from build123d import *

# Parameters (mm, degrees)
SCHIZZO13_R                  = 1.5
SCHIZZO13_R_2                = 2.75
SCHIZZO13_R_3                = 1.25
ESTRUSIONE_ESTRUSIONE2_DEPTH = 6


with BuildPart() as part:
    # Schizzo13 → Estrusione-Estrusione2 (new body)
    with BuildSketch(Plane.XY):
        with BuildLine():
            Line((9.919241786, 0), (24.201199756, 0))
            Line((24.201199756, 0), (34.201199756, 10))
            Line((34.201199756, 10), (34.28195797, 30))
            Line((34.28195797, 30), (57.017366293, 53.192694567))
            Line((57.017366293, 53.192694567), (83.745372993, 53.192694567))
            Line((83.745372993, 53.192694567), (107.404551383, 30))
            Line((107.404551383, 30), (107.404551383, 10))
            Line((107.404551383, 10), (117.404551383, 0))
            Line((117.404551383, 0), (232.595448617, 0))
            Line((232.595448617, 0), (242.595448617, 10))
            Line((242.595448617, 10), (242.595448617, 30))
            Line((242.595448617, 30), (266.254627007, 53.192694567))
            Line((266.254627007, 53.192694567), (292.982633707, 53.192694567))
            Line((292.982633707, 53.192694567), (315.71804203, 30))
            Line((315.71804203, 30), (315.71804203, 10))
            Line((315.71804203, 10), (325.71804203, 0))
            Line((325.71804203, 0), (340, 0))
            Line((340, 0), (350, 10))
            Line((350, 10), (350.080758214, 70.5))
            Line((350.080758214, 70.5), (293, 124.388863529))
            Line((293, 124.388863529), (293, 225.611136471))
            Line((293, 225.611136471), (350.080758214, 279.5))
            Line((350.080758214, 279.5), (350, 340))
            Line((350, 340), (340, 350))
            Line((340, 350), (302.982633707, 350))
            Line((302.982633707, 350), (292.982633707, 340))
            Line((292.982633707, 340), (292.982633707, 299.807305433))
            ThreePointArc((292.982633707, 299.807305433), (292.103954051, 297.685985089), (289.982633707, 296.807305433))
            Line((289.982633707, 296.807305433), (266.254627007, 296.807305433))
            Line((266.254627007, 296.807305433), (242.595448617, 320))
            Line((242.595448617, 320), (242.595448617, 340))
            Line((242.595448617, 340), (232.595448617, 350))
            Line((232.595448617, 350), (117.404551383, 350))
            Line((117.404551383, 350), (107.404551383, 340))
            Line((107.404551383, 340), (107.404551383, 320))
            Line((107.404551383, 320), (83.745372993, 296.807305433))
            Line((83.745372993, 296.807305433), (57.017366293, 296.807305433))
            Line((57.017366293, 296.807305433), (34.28195797, 320))
            Line((34.28195797, 320), (34.28195797, 340))
            Line((34.28195797, 340), (24.201199756, 350))
            Line((24.201199756, 350), (9.919241786, 350))
            Line((9.919241786, 350), (-0.080758214, 340))
            Line((-0.080758214, 340), (-0.080758214, 279.5))
            Line((-0.080758214, 279.5), (57, 225.611136471))
            Line((57, 225.611136471), (57, 175))
            Line((57, 175), (57, 124.388863529))
            Line((57, 124.388863529), (-0.080758214, 70.5))
            Line((-0.080758214, 70.5), (-0.080758214, 10))
            Line((-0.080758214, 10), (9.919241786, 0))
        make_face()
        with Locations((15, 320)):
            Circle(SCHIZZO13_R, mode=Mode.SUBTRACT)
        with Locations((20.5, 279.5)):
            Circle(SCHIZZO13_R, mode=Mode.SUBTRACT)
        with Locations((70.5, 279.5)):
            Circle(SCHIZZO13_R, mode=Mode.SUBTRACT)
        with Locations((175, 175)):
            Circle(SCHIZZO13_R, mode=Mode.SUBTRACT)
        with Locations((20.5, 70.5)):
            Circle(SCHIZZO13_R, mode=Mode.SUBTRACT)
        with Locations((200, 344)):
            Circle(SCHIZZO13_R_2, mode=Mode.SUBTRACT)
        with Locations(Location((150, 344, 0), (0, 0, 180))):
            Circle(SCHIZZO13_R_2, mode=Mode.SUBTRACT)
        with Locations((175, 329)):
            Circle(SCHIZZO13_R_2, mode=Mode.SUBTRACT)
        with Locations((217, 329)):
            Circle(SCHIZZO13_R_2, mode=Mode.SUBTRACT)
        with Locations(Location((133, 329, 0), (0, 0, 180))):
            Circle(SCHIZZO13_R_2, mode=Mode.SUBTRACT)
        with Locations((70.5, 70.5)):
            Circle(SCHIZZO13_R, mode=Mode.SUBTRACT)
        with Locations((279.5, 70.5)):
            Circle(SCHIZZO13_R, mode=Mode.SUBTRACT)
        with Locations((329.5, 70.5)):
            Circle(SCHIZZO13_R, mode=Mode.SUBTRACT)
        with Locations((335, 10)):
            Circle(SCHIZZO13_R, mode=Mode.SUBTRACT)
        with Locations((15, 10)):
            Circle(SCHIZZO13_R, mode=Mode.SUBTRACT)
        with Locations((279.5, 279.5)):
            Circle(SCHIZZO13_R, mode=Mode.SUBTRACT)
        with Locations((329.5, 279.5)):
            Circle(SCHIZZO13_R, mode=Mode.SUBTRACT)
        with Locations((335, 320)):
            Circle(SCHIZZO13_R, mode=Mode.SUBTRACT)
        with Locations((310, 344)):
            Circle(SCHIZZO13_R, mode=Mode.SUBTRACT)
        with Locations((330, 344)):
            Circle(SCHIZZO13_R, mode=Mode.SUBTRACT)
        with Locations((122.656966622, 15)):
            Circle(SCHIZZO13_R_3, mode=Mode.SUBTRACT)
        with Locations(Location((227.343033378, 15, 0), (0, 0, 180))):
            Circle(SCHIZZO13_R_3, mode=Mode.SUBTRACT)
        Polygon((217, 193.286910978), (227.343033378, 225.611136471), (185.750894453, 266.383210572), (164.249105547, 266.383210572), (122.656966622, 225.611136471), (133, 193.286910978), align=None, mode=Mode.SUBTRACT)
        Polygon((133, 156.713089022), (101.348199345, 83.616789428), (155.254193112, 30), (194.745806888, 30), (248.651800655, 83.616789428), (217, 156.713089022), align=None, mode=Mode.SUBTRACT)
    extrude(amount=-ESTRUSIONE_ESTRUSIONE2_DEPTH)


solid = part.part
Source: CAD feature listing. Evaluate the final solid. Frame: model axes, mm. A direction names the side the tool comes from. Round coordinates to 2 decimals unless told otherwise and drop trailing zeros. Loops run counter-clockwise (first coordinate to the right, second up) from the corner with the lowest first, then second, coordinate; pieces in that order, holes last. Notation, with made-up numbers: M 88.5,59.25 L 122.5,59.25 A21 cw 122.5,76.25 Z; hole C 77.5,68 d8. An arc over 180 degrees is marked long. Answer as CSV lines item,"result".
Q1. Reachability of faces 1 (the face through (237.665, 344.93, -2.958)), 2 (the face through (95.41, 41.76, -2.96)), 3 (the face through (321.14, 252.18, -2.96)), 4 (the face through (117.396, 120.677, -2.958)) from +Z, -Z, +X, -X, +Y, -Y: full face, straight path, thin tool, end or side. Return the list, or none.
Verdict:
face 1,"+Z, -Z, +Y"
face 2,"+Z, -Z, -Y"
face 3,"+Z, -Z, +X"
face 4,"+Z, -Z"
Q2. Cut plane B-B (x = 49). Return the cut outline in (y, z).
Verdict:
outline,"M 45.01,-6 L 116.84,-6 L 116.84,0 L 45.01,0 Z; M 233.16,-6 L 304.99,-6 L 304.99,0 L 233.16,0 Z"
Q3. Line query: line 1 along Y through (x, z) = (70.5, -1.4); line 2 along X through (y, z) = (329, -2.85); line 3 along X through (y, z) = (279.5, -3.1). Output: solid intervals per line, ascending.
Verdict:
line 1,"y = 53.19 to 69, 72 to 278, 281 to 296.81"
line 2,"x = -0.08 to 34.28, 107.4 to 130.25, 135.75 to 172.25, 177.75 to 214.25, 219.75 to 242.6, 292.98 to 350.01"
line 3,"x = -0.08 to 19, 22 to 69, 72 to 278, 281 to 328, 331 to 350.08"
Q4. Cut plane C-C (z = -2.75). Count the separate pieces of the cut face and the enclosed holes in it, plus the area to 3 significant figures.
Verdict:
separate pieces,"1"
enclosed holes,"24"
area,"72,500 mm^2"
Q5. Cut plane A-A (y = 144). Return the cut outline in (x, z), plus the area to 3 significant figures.
Verdict:
outline,"M 57,-6 L 127.5,-6 L 127.5,0 L 57,0 Z; M 222.5,-6 L 293,-6 L 293,0 L 222.5,0 Z"
area,"846 mm^2"
Q6. Contact query for flat-ended pins moving along their axis: pin 1 (2 mm diameter, centred on x = 109, z = -1, fed in from -Y); pin 2 (1 mm diameter, centred on y = 173, z = -5, fed in from +X); pin 3 (3 mm diameter, centred on x = 73.5, z = -3, fed in from -Y). Output: stop coordinate, or through.
Verdict:
pin 1,"stops at y = 7.4"
pin 2,"stops at x = 293"
pin 3,"stops at y = 53.19"
Q7. Pull-direction query (X, two-part tool) for faces 5 (the face through (127.924, 57.184, -2.958)), 6 (the face through (321.94, 97.067, -2.958)), 7 (the face through (28.86, 97.82, -2.96)); classes: +X half, -X half, draft (parallel to the pull), parting line (faces both ways), or undercut.
Verdict:
face 5,"undercut"
face 6,"+X half"
face 7,"-X half"
